Here's how the part is built. I have some questions about the finished solid (model axes, mm). Face numbers are marked on the shaded views. A direction names the side the tool comes from. Give positions to 0.01 mm unless a question says otherwise; leave off trailing zeros. Order: outer loops, then holes, each group sorted by start corner. A loop starts at its lowest first (then second) coordinate and runs counter-clockwise, first axis right, second up.
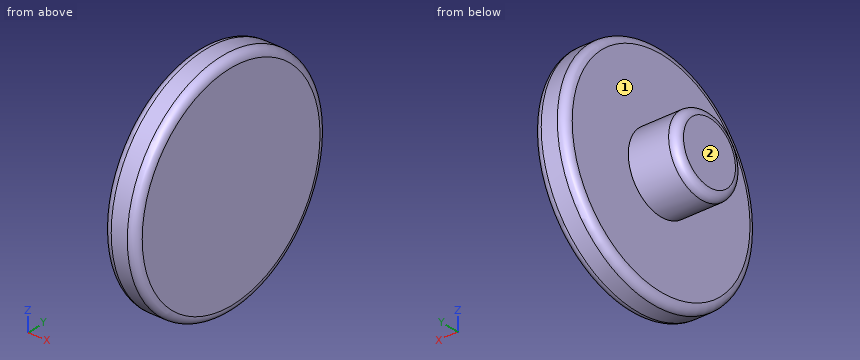
from build123d import *

# Parameters (mm, degrees)
F0_R     = 7
F0_R_2   = 2.4
F1_DEPTH = 2
F2_DEPTH = 3
F3_R     = 0.5


with BuildPart() as f1:
    # F0 (on Right) → F1 (new body)
    with BuildSketch(Plane.YZ):
        Circle(F0_R)
        Circle(F0_R_2, mode=Mode.SUBTRACT)
        Circle(F0_R_2)
    extrude(amount=F1_DEPTH)

    # F0 (on Right) → F2 (join)
    with BuildSketch(Plane.YZ):
        Circle(F0_R_2)
    extrude(amount=-F2_DEPTH)

    # F3
    f3_edges = [f1.edges().sort_by_distance(p)[0] for p in [
        (2, -7, 0),
        (-3, -2.4, 0),
        (0, -7, 0),
    ]]
    fillet(f3_edges, radius=F3_R)


solid = f1.part
Q1. For the marked faces 1 and 2, which set-ups out of +Z, -Z, +X, -X, +Y, -Y let a thin tool reach every point of the face, with its end or its side?
Filled sheet:
face 1: -X
face 2: +Z, -Z, -X, +Y, -Y
Q2. I need wall thicknesses on L1, parallel to X at y = -2, z = -5.25; L2, parallel to Y at x = 0.1, z = 4.75; L3, parallel to Z at x = 0.2, y = -4.5. Which ranges of each line are inside material? Lowest first, please.
Filled sheet:
L1: x = 0 to 2
L2: y = -4.87 to 4.87
L3: z = -5.23 to 5.23
Q3. If we section it at C-C on x = 0.2: List the corners of the cut face in (y, z) for me.
Filled sheet:
outline: circle Ø13.8 at (0, 0)
Q4. I'm going to push flat-ended pins straight in: P1, Ø1.5, axis at x = -2.5, y = -4.5, coming from the -Z side; P2, Ø2, axis at x = 0.5, y = -5.5, coming from the -Z side; P3, Ø3, axis at y = -1.5, z = 3, coming from the -X side. Where does each tip first touch, or does it pass through?
Filled sheet:
P1: passes through
P2: stops at z = -5.36
P3: stops at x = -3
Q5. If we section it at A-A on z = 0: List the corners of the cut face in (x, y) for me.
Filled sheet:
outline: (-3, -1.9) arc R0.5 ccw to (-2.5, -2.4) - (0, -2.4) - (0, -6.5) arc R0.5 ccw to (0.5, -7) - (1.5, -7) arc R0.5 ccw to (2, -6.5) - (2, 6.5) arc R0.5 ccw to (1.5, 7) - (0.5, 7) arc R0.5 ccw to (0, 6.5) - (0, 2.4) - (-2.5, 2.4) arc R0.5 ccw to (-3, 1.9) - close
